Check sheet for the modelled part. Datum: model origin and axes. Units: mm. A direction names the side the tool comes from. Give positions to 0.01 mm unless a question says otherwise; leave off trailing zeros. Loops run counter-clockwise (first coordinate to the right, second up) from the corner with the lowest first, then second, coordinate; pieces in that order, holes last. Notation, with made-up numbers: (51, 32.5) - (100, 32.5) arc R16 cw to (100, 42.5) - close; hole circle Ø1 at (72, -10.5). An arc over 180 degrees is marked (long way). Use one line per item in the form item = value.
from build123d import *

# Parameters (mm, degrees)
SKETCH1_R                = 150
BOSS_EXTRUDE1_DEPTH      = 50
BOSS_EXTRUDE2_DEPTH      = 10
BOSS_EXTRUDE2_DEPTH_BACK = 60
SKETCH3_R                = 2.5
CUT_EXTRUDE1_DEPTH       = 10


with BuildPart() as part:
    # Sketch1 → Boss-Extrude1 (new body)
    with BuildSketch(Plane.XY):
        Circle(SKETCH1_R)
        with BuildLine():
            Line((-7, 22.5), (7, 22.5))
            Line((7, 22.5), (7, 16.039014932))
            ThreePointArc((7, 16.039014932), (0, -17.5), (-7, 16.039014932))
            Line((-7, 16.039014932), (-7, 22.5))
        make_face(mode=Mode.SUBTRACT)
    extrude(amount=BOSS_EXTRUDE1_DEPTH)

    # Sketch2 → Boss-Extrude2 (add, two sides: drawn at the far end of the back side and taken through both)
    with BuildSketch(Plane.XY.offset(50).offset(-BOSS_EXTRUDE2_DEPTH_BACK)):
        with BuildLine():
            Line((17, 21.615966321), (17, 32.5))
            Line((17, 32.5), (-17, 32.5))
            Line((-17, 32.5), (-17, 21.615966321))
            ThreePointArc((-17, 21.615966321), (0, -27.5), (17, 21.615966321))
        make_face()
        with BuildLine():
            Line((7, 16.039014932), (7, 22.5))
            Line((7, 22.5), (-7, 22.5))
            Line((-7, 22.5), (-7, 16.039014932))
            ThreePointArc((-7, 16.039014932), (0, -17.5), (7, 16.039014932))
        make_face(mode=Mode.SUBTRACT)
    extrude(amount=BOSS_EXTRUDE2_DEPTH + BOSS_EXTRUDE2_DEPTH_BACK)

    # Sketch3 → Cut-Extrude1 (cut)
    with BuildSketch(Plane(origin=(0, 32.5, 0), x_dir=(1, 0, 0), z_dir=(0, 1, 0))):
        with Locations(Location((0, -55, 0), (0, 0, 270))):
            Circle(SKETCH3_R)
    extrude(amount=-CUT_EXTRUDE1_DEPTH, mode=Mode.SUBTRACT)


solid = part.part
Item 1: Section check D-D on y = 43. Record the boundary of the cut face in (x, z).
Answer block:
outline = (-143.7, 0) - (143.7, 0) - (143.7, 50) - (-143.7, 50) - close
Item 2: Thickness scan on L1, parallel to Y at x = 0, z = 15.5; L2, parallel to X at y = 28, z = 55; L3, parallel to Z at x = -71, y = 90. Record the ranges inside material, lowest first.
Answer block:
L1 = -150 to -17.5, 22.5 to 150
L2 = -17 to -2.5, 2.5 to 17
L3 = 0 to 50
Item 3: Section check B-B on z = 4. Record the boundary of the cut face in (x, y), then the cut area to 3 significant figures.
Answer block:
outline = circle Ø300 at (0, 0); hole (-7, 16.04) arc R17.5 ccw (long way) to (7, 16.04) - (7, 22.5) - (-7, 22.5) - close
area = 69,600 mm2
Item 4: Access from +Z, -Z, +X, -X, +Y, -Y to the whole of each face (thin tool, end or side, straight path). Record for faces 1 (the face through (-7, 19, 25)), 2 (the face through (0, 32.5, 58)), 3 (the face through (-17, 27, -5)), 4 (the face through (0, 32.5, -5)), 5 (the face through (-0.953, -27.483, 54.93)).
Answer block:
face_1 = +Z, -Z
face_2 = +Z, +X, -X, +Y
face_3 = -Z, -X, +Y
face_4 = -Z, +X, -X, +Y
face_5 = +Z
Item 5: Section check C-C on x = -43.5. Record the boundary of the cut face in (y, z), then the cut area to 3 significant figures.
Answer block:
outline = (-143.55, 0) - (143.55, 0) - (143.55, 50) - (-143.55, 50) - close
area = 14,400 mm2
Item 6: Section check A-A on y = 0. Record the boundary of the cut face in (x, z), then the cut area to 4 significant figures.
Answer block:
outline = (-150, 0) - (-27.5, 0) - (-27.5, -10) - (-17.5, -10) - (-17.5, 60) - (-27.5, 60) - (-27.5, 50) - (-150, 50) - close; (17.5, -10) - (27.5, -10) - (27.5, 0) - (150, 0) - (150, 50) - (27.5, 50) - (27.5, 60) - (17.5, 60) - close
area = 13,650 mm2
Item 7: Mould release check, pull along Y, two halves, no side actions. Record for faces 6 (the face through (17, 27, -5)), 7 (the face through (-0.953, -27.483, -5.07)), 8 (the face through (-0.669, -17.487, 24.51)), 9 (the face through (0, 22.5, 25)): released by +Y, released by -Y, zero draft, split by the parting line, or undercut.
Answer block:
face_6 = zero draft
face_7 = split by the parting line
face_8 = undercut
face_9 = undercut
Item 8: Gauge pin test, flat ends, axial feed: P1, Ø5, axis at x = -75, z = 33, coming from the -Y side; P2, Ø5, axis at x = 4, z = 54, coming from the +Y side; P3, Ø11, axis at y = 25.5, z = -6, coming from the +X side; P4, Ø21, axis at x = 0, y = 0, coming from the +Z side. Record the tip position at first contact, or that the pin passes through.
Answer block:
P1 = -131.32
P2 = 32.5
P3 = 18.87
P4 = through
